Model file for the job. Use its own axes, mm. Face numbers are marked on the shaded views. A direction names the side the tool comes from. Coordinates: 2 decimals unless noted, no trailing zeros. Write each loop counter-clockwise with the first axis right and the second up, starting at its lowest first coordinate (ties: lowest second). Pieces come first, ordered by that corner, then holes. Notation, with made-up numbers: M 73,79 L 106,79 A20 cw 106,113 Z; hole C 54.25,24.25 d9. An arc over 180 degrees is marked long. Put each result on its own line as item: value. Start each with the question number.
Q1. Pull direction Z, two halves, no side cores. Call the marked faces 5, 6 and 7: pulls with the +Z half, pulls with the -Z half, needs draft (parallel to the pull), parting line crosses it, or undercut.
Q2. Cut at D-D (x = -15). Write the cut outline in (y, z).
Q3. Which spindle directions (+Z, -Z, +X, -X, +Y, -Y) get a long thin tool onto all of the face, cutting with end or side? Do the marked faces 1, 2, 3 and 4. Say none if no direction does.
Q4. Cut at B-B (y = 6.5). Write the cut outline in (x, z).
Q5. Cut at C-C (z = -19.5). Write the cut outline in (x, y).
Q6. Drop flat-ended pins along their axis: pin 1 (1.4 mm diameter, centred on y = 3, z = -30, fed in from +X); pin 2 (10 mm diameter, centred on y = 11, z = -26, fed in from +X); pin 3 (1.6 mm diameter, centred on x = -13.5, z = -3.5, fed in from +Y); pin 4 (0.8 mm diameter, centred on y = 4, z = -35.5, fed in from -X). Give the stop position or say it passes through.
Q7. Drill centre lines: line 1 along X through (y, z) = (1.6, -30.7) (3 decimals); line 2 along Z through (x, y) = (-23, 1.35) (3 decimals); line 3 along Z through (x, y) = (-17, 4). Where is each one in solid material? Low to high.
Q8. Cut at A-A (x = -23). Write the cut outline in (y, z) (3 decimals).
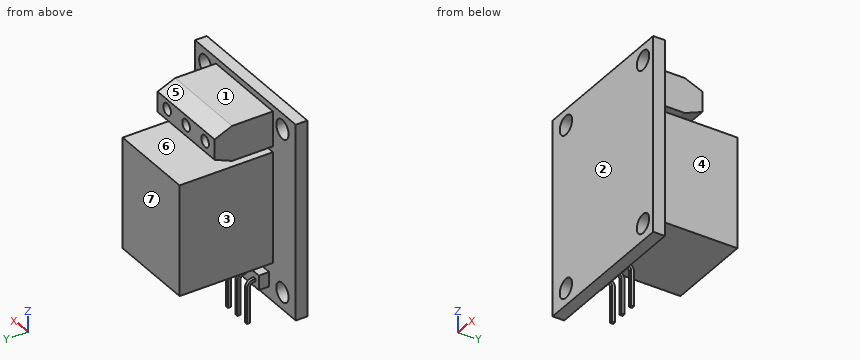
Autodesk Inventor part; units mm, degrees
ref_plane "YZ Plane" through (0, 0, 0) normal (1, 0, 0) x (0, 1, 0)
ref_plane "XZ Plane" through (0, 0, 0) normal (0, 1, 0) x (-1, 0, 0)
ref_plane "XY Plane" through (0, 0, 0) normal (0, 0, 1) x (1, 0, 0)
sketch "Sketch1" plane through (0, 0, 0) normal (0, 1, 0) x (-1, 0, 0)
  line L0 (0, 0) -> (26.5, 0)
  line L1 (26.5, 0) -> (26.5, -33.6)
  line L2 (26.5, -33.6) -> (0, -33.6)
  line L3 (0, -33.6) -> (0, 0)
  dimension "d0" = 33.6
  dimension "d1" = 26.5
extrude "Extrusion1" add sketch "Sketch1" along normal blind 2
sketch "Sketch2" plane through (0, 2, 0) normal (0, 1, 0) x (1, 0, 0)
  line L0 (-20.5, 8) -> (-5.5, 8)
  line L1 (-5.5, 8) -> (-5.5, 27)
  line L2 (-5.5, 27) -> (-20.5, 27)
  line L3 (-20.5, 27) -> (-20.5, 8)
  line L4 (-26.5, 0) -> (0, 0) construction
  line L5 (0, 0) -> (0, 33.6) construction
  line L6 (0, 33.6) -> (-26.5, 33.6) construction
  line L7 (-26.5, 33.6) -> (-26.5, 0) construction
  line L8 (-20.5, 8) -> (-26.5, 8) construction
  line L9 (-26.5, 33.6) -> (-26.5, 0) construction
  line L10 (-5.5, 8) -> (0, 8) construction
  dimension "d4" = 15
  dimension "d5" = 19
  dimension "d6" = 8
  dimension "d36" = 5.5
extrude "Extrusion2" add sketch "Sketch2" along normal blind 16
sketch "Sketch3" plane through (0, 2, 0) normal (0, 1, 0) x (1, 0, 0)
  line L0 (-12, 31.6) -> (-19.5, 31.6)
  line L1 (-19.5, 31.6) -> (-19.5, 29.1)
  line L2 (-19.5, 29.1) -> (-12, 29.1)
  line L3 (-12, 29.1) -> (-12, 31.6)
  line L4 (-19.5, 29.1) -> (-26.5, 29.1) construction
  line L5 (-26.5, 33.6) -> (-26.5, 0) construction
  line L6 (-12, 29.1) -> (-5, 29.1) construction
  line L7 (0, 33.6) -> (-26.5, 33.6) construction
  line L8 (-13.625, 30.1) -> (-13.125, 30.1)
  line L9 (-13.125, 30.1) -> (-13.125, 30.6)
  line L10 (-13.125, 30.6) -> (-13.625, 30.6)
  line L11 (-13.625, 30.6) -> (-13.625, 30.1)
  line L12 (-16.125, 30.1) -> (-15.625, 30.1)
  line L13 (-15.625, 30.1) -> (-15.625, 30.6)
  line L14 (-15.625, 30.6) -> (-16.125, 30.6)
  line L15 (-16.125, 30.6) -> (-16.125, 30.1)
  line L16 (-18.625, 30.1) -> (-18.125, 30.1)
  line L17 (-18.125, 30.1) -> (-18.125, 30.6)
  line L18 (-18.125, 30.6) -> (-18.625, 30.6)
  line L19 (-18.625, 30.6) -> (-18.625, 30.1)
  line L20 (-13.125, 30.1) -> (-13.125, 29.1) construction
  line L21 (-13.125, 30.6) -> (-13.125, 31.6) construction
  point P0 (0, 0)
  dimension "d9" = 2
  dimension "d10" = 2.5
  dimension "d11" = 7.5
  dimension "d12" = 0.5
  dimension "d13" = 0.5
  dimension "d16" = 2.5
  dimension "d21" = 1.125
  dimension "d39" = 7
extrude "Extrusion3" add sketch "Sketch3" along normal blind 1.75
sketch "Sketch4" plane through (-5.5, 2, -8) normal (1, 0, 0) x (0, 0, -1)
  line L0 (-8, 0) -> (25.6, 0) construction
  line L1 (0, 0) -> (0, 16) construction
  line L2 (-1, 0) -> (-1, 7)
  line L3 (-1, 7) -> (-2.25, 10)
  line L4 (-2.25, 10) -> (-5.75, 10)
  line L5 (-5.75, 10) -> (-7, 7)
  line L6 (-7, 7) -> (-7, 0)
  line L7 (25.6, 0) -> (-8, 0)
  line L8 (-7, 0) -> (-1, 0)
  line L9 (-8, -2) -> (-8, 0)
  dimension "d26" = 6
  dimension "d27" = 10
  dimension "d28" = 3
  dimension "d37" = 1
  dimension "d38" = 3.5
extrude "Extrusion5" add sketch "Sketch4" against normal up to surface (15 mm away)
sketch "Sketch5" plane through (-5.5, 12, -2.25) normal (0, 1, 0) x (1, 0, 0)
  line L0 (0, 0) -> (-15, 0) construction
  circle A0 centre (-2.5, 1.6688) radius 1
  circle A1 centre (-7.5, 1.6688) radius 1
  circle A2 centre (-12.5, 1.6688) radius 1
  line L1 (-12.5, 1.6688) -> (-15, 1.6688) construction
  line L2 (-2.5, 1.6688) -> (0, 1.6688) construction
  line L3 (-15, 3.5) -> (-15, 0) construction
  line L4 (0, 3.5) -> (0, 0) construction
  point P0 (5.5, -2.25)
  dimension "d31" = 2
  dimension "d32" = 5
  dimension "d33" = 5
extrude "Extrusion6" cut sketch "Sketch5" against normal blind 1
sketch "Sketch6" plane through (-12, 2, -29.1) normal (1, 0, 0) x (0, 0, -1)
  line L0 (-29.1, 0) -> (4.5, 0) construction
  line L1 (2.5, 0) -> (2.5, 1.75) construction
  line L2 (0, 0) -> (0, 1.75) construction
  line L3 (1, 0) -> (1.5, 0)
  line L4 (1.25, 0) -> (1.25, 2)
  arc A0 (2.25, 3) -> (1.25, 2) centre (2.25, 2) ccw
  line L5 (2.25, 3) -> (8.25, 3)
  point P0 (-29.1, -2)
  dimension "d40" = 2
  dimension "d41" = 6
  dimension "d42" = 1
sweep "Sweep1" add profiles "Sketch3" path "Sketch6" path curves L4 A0 L5 contours L11 L10 L9 L8 | L15 L14 L13 L12 | L19 L18 L17 L16
hole "Hole1" at (-2.7, 2, -2.7) direction (0, -1, 0) diameter 3.25 end through all
pattern_linear "Rectangular Pattern1" count 2 spacing 20.3 along (-1, 0, 0) count 2 spacing 28 along (0, 0, -1) of "Hole1"
properties part number "RelayModule" material "ABS Plastic"
Computed values:
1. face 5: pulls with the +Z half
1. face 6: undercut
1. face 7: needs draft
2. outline: M 0,-33.6 L 2,-33.6 L 2,-31.6 L 3.75,-31.6 L 3.75,-29.1 L 2,-29.1 L 2,-27 L 18,-27 L 18,-8 L 2,-8 L 2,-7 L 9,-7 L 12,-5.75 L 12,-2.25 L 9,-1 L 2,-1 L 2,0 L 0,0 Z
3. face 1: +Z, +X, -X, +Y
3. face 2: +Z, -Z, +X, -X, -Y
3. face 3: +Z, -Z, -X, +Y
3. face 4: +Z, -Z, +X, +Y
4. outline: M -20.5,-27 L -5.5,-27 L -5.5,-8 L -20.5,-8 Z; M -20.5,-7 L -5.5,-7 L -5.5,-1 L -20.5,-1 Z
5. outline: M -26.5,0 L 0,0 L 0,2 L -5.5,2 L -5.5,18 L -20.5,18 L -20.5,2 L -26.5,2 Z
6. pin 1: x = -12
6. pin 2: x = -5.5
6. pin 3: y = 12
6. pin 4: through
7. line 1: -26.5 to -24.625, -21.375 to -4.325, -1.075 to 0
7. line 2: -33.6 to -32.325, -29.075 to -4.325, -1.075 to 0
7. line 3: -27 to -8, -7 to -1
8. outline: M 0,-33.6 L 2,-33.6 L 2,-32.325 L 0,-32.325 Z; M 0,-29.075 L 2,-29.075 L 2,-4.325 L 0,-4.325 Z; M 0,-1.075 L 2,-1.075 L 2,0 L 0,0 Z
